Here's how the part is built. I have some questions about the finished solid (model axes, mm). Coordinates: 2 decimals unless noted, no trailing zeros. Write each loop counter-clockwise with the first axis right and the second up, starting at its lowest first coordinate (ties: lowest second). Pieces come first, ordered by that corner, then holes.
(1) Please list where these lines run through material, in increasing order: probe 1 along Y at (x, z) = (44.5, 22); probe 2 along X at (y, z) = (-10.5, -48); probe 3 along Z at (x, y) = (0, -31.5).
(2) Imagine slicing it at C-C, the plane y = -29.5. List the corners of the cut face in (x, z) for me, plus the area to 3 significant figures.
(3) For pin 1 Ø23 at (x, z) = (-65.99, -38.1) entering from -Y; pin 2 Ø10 at (x, y) = (-21.5, -48.5) entering from +Z; pin 3 Ø10 at (y, z) = (-53.5, -35) entering from +X, each with a flat end and sliding along its axis, tell me the tip position at first contact or that it passes through.
(4) Imagine slicing it at D-D, the plane z = 0. List the corners of the cut face in (x, y) for me, plus the area to 3 significant figures.
(5) Imagine slicing it at A-A, the plane x = 63. List the corners of the cut face in (y, z) for me.
(6) Thinking about a two-plate mould opening in Z: for faces 1 (the flat face through (44, -50.8, 1)), 2 (the cylindrical face through (53.303, -25.756, -37.542)), 3 (the cylindrical face through (-30.235, -75.844, -23.183)), which applies, released by +Z, released by -Z, zero draft, split by the parting line, or undercut?
(7) Imagine slicing it at B-B, the plane z = 76.2. List the corners of the cut face in (x, y) for me, plus the area to 3 significant figures.
```python
from build123d import *

# Parameters (mm, degrees)
F0_R     = 101.6
F1_DEPTH = 50.8
F2_R     = 38.1
F3_DEPTH = 50.8
F4_R     = 12.7
F5_DEPTH = 87.376


with BuildPart() as f1:
    # F0 (on Front) → F1 (new body)
    with BuildSketch(Plane.XZ):
        Circle(F0_R)
    extrude(amount=F1_DEPTH)

    # F2 (on face) → F3 (join)
    with BuildSketch(Plane.XZ.offset(50.8)):
        Circle(F2_R)
    extrude(amount=F3_DEPTH)

    # F4 (on face) → F5 (cut)
    with BuildSketch(Plane.XZ.offset(50.8)):
        with Locations((0, 76.2)):
            Circle(F4_R)
        with Locations((-65.991136, -38.1)):
            Circle(F4_R)
        with Locations((65.991136, -38.1)):
            Circle(F4_R)
    extrude(amount=-F5_DEPTH, mode=Mode.SUBTRACT)


solid = f1.part
```
Recorded:
1. probe 1: y = -50.8 to 0
1. probe 2: x = -89.55 to -73.95, -58.04 to 58.04, 73.95 to 89.55
1. probe 3: z = -101.6 to 63.5, 88.9 to 101.6
2. outline: circle Ø203.2 at (0, 0); hole circle Ø25.4 at (-65.99, -38.1); hole circle Ø25.4 at (0, 76.2); hole circle Ø25.4 at (65.99, -38.1)
2. area: 30,900 mm2
3. pin 1: passes through
3. pin 2: stops at z = 100.25
3. pin 3: stops at x = 96.82
4. outline: (-101.6, -50.8) - (-38.1, -50.8) - (-38.1, -101.6) - (38.1, -101.6) - (38.1, -50.8) - (101.6, -50.8) - (101.6, 0) - (-101.6, 0) - close
4. area: 14,200 mm2
5. outline: (-50.8, -79.71) - (0, -79.71) - (0, -50.44) - (-50.8, -50.44) - close; (-50.8, -25.76) - (0, -25.76) - (0, 79.71) - (-50.8, 79.71) - close
6. face 1: zero draft
6. face 2: undercut
6. face 3: split by the parting line
7. outline: (-67.2, -50.8) - (-12.7, -50.8) - (-12.7, 0) - (-67.2, 0) - close; (12.7, -50.8) - (67.2, -50.8) - (67.2, 0) - (12.7, 0) - close
7. area: 5,540 mm2
